from build123d import *

# Parameters (mm, degrees)
SKETCH1_R           = 1.85
SKETCH1_W           = 4.8
SKETCH1_H           = 4.8
BOSS_EXTRUDE1_DEPTH = 1.57
SKETCH2_W           = 4.8
SKETCH2_H           = 4.8
BOSS_EXTRUDE2_DEPTH = 1.47


with BuildPart() as part:
    # Sketch1 → Boss-Extrude1 (new body)
    # profile 1 of 2: a face of its own
    with BuildSketch(Plane(origin=(0, 0, 0), x_dir=(1, 0, 0), z_dir=(0, 1, 0))):
        with BuildLine():
            ThreePointArc((-11.5, 9.5), (-10.914213562, 10.914213562), (-9.5, 11.5))
            Line((-9.5, 11.5), (9.5, 11.5))
            ThreePointArc((9.5, 11.5), (10.914213562, 10.914213562), (11.5, 9.5))
            Line((11.5, 9.5), (11.5, -9.5))
            ThreePointArc((11.5, -9.5), (10.914213562, -10.914213562), (9.5, -11.5))
            Line((9.5, -11.5), (-9.5, -11.5))
            ThreePointArc((-9.5, -11.5), (-10.914213562, -10.914213562), (-11.5, -9.5))
            Line((-11.5, -9.5), (-11.5, 9.5))
        make_face()
        with Locations(Location((-8, -8, 0), (0, 0, 270))):
            Circle(SKETCH1_R, mode=Mode.SUBTRACT)
        with Locations(Location((8, -8, 0), (0, 0, 270))):
            Circle(SKETCH1_R, mode=Mode.SUBTRACT)
        with Locations(Location((8, 8, 0), (0, 0, 270))):
            Circle(SKETCH1_R, mode=Mode.SUBTRACT)
        with Locations(Location((-8, 8, 0), (0, 0, 270))):
            Circle(SKETCH1_R, mode=Mode.SUBTRACT)
        Rectangle(SKETCH1_W, SKETCH1_H, mode=Mode.SUBTRACT)
    # profile 2 of 2: a face of its own
    with BuildSketch(Plane(origin=(0, 0, 0), x_dir=(1, 0, 0), z_dir=(0, 1, 0))):
        Rectangle(SKETCH1_W, SKETCH1_H)
    extrude(amount=BOSS_EXTRUDE1_DEPTH)

    # Sketch2 → Boss-Extrude2 (add)
    with BuildSketch(Plane(origin=(0, 1.57, 0), x_dir=(1, 0, 0), z_dir=(0, 1, 0))):
        Rectangle(SKETCH2_W, SKETCH2_H)
    extrude(amount=BOSS_EXTRUDE2_DEPTH)


solid = part.part
Geometry check sheet. Reference: the model listing, model coordinates, mm. A direction names the side the tool comes from. Coordinates: 2 decimals unless noted, no trailing zeros. Order: outer loops, then holes, each group sorted by start corner. A loop starts at its lowest first (then second) coordinate and runs counter-clockwise, first axis right, second up. Notation, with made-up numbers: M 23,-11 L 39,-11 A28 ccw 39,23 Z; hole C 46.25,26 d4. An arc over 180 degrees is marked long. Use CSV: the item, a comma, the result in double quotes.
Item 1: Cross-section at D-D on x = 1.5. Record the cut outline in (y, z).
Returned:
outline,"M 0,-11.5 L 1.57,-11.5 L 1.57,-2.4 L 3.04,-2.4 L 3.04,2.4 L 1.57,2.4 L 1.57,11.5 L 0,11.5 Z"
Item 2: Tool access check on faces 4 (the flat face through (-2.4, 2, 0)), 5 (the flat face through (0, 2, -2.4)), 6 (the flat face through (0, 2, 2.4)), 7 (the flat face through (2.4, 2, 0)). Record the directions out of +Z, -Z, +X, -X, +Y, -Y that give a thin tool (end or side, any length) a straight path to the whole face; none if there is none.
Returned:
face 4,"+Z, -Z, -X, +Y"
face 5,"-Z, +X, -X, +Y"
face 6,"+Z, +X, -X, +Y"
face 7,"+Z, -Z, +X, +Y"
Item 3: Mould release check, pull along X, two halves, no side actions. Record for faces 1 (the cylindrical face through (6.874, 0.774, 6.532)), 2 (the flat face through (0, 1.57, -3)), 3 (the flat face through (-11.5, 1, 0)): pulls with the +X half, pulls with the -X half, needs draft (parallel to the pull), parting line crosses it, or undercut.
Returned:
face 1,"undercut"
face 2,"needs draft"
face 3,"pulls with the -X half"
Item 4: Cross-section at B-B on x = 8. Record the cut outline in (y, z), then the cut area to 3 significant figures.
Returned:
outline,"M 0,-11.5 L 1.57,-11.5 L 1.57,-9.85 L 0,-9.85 Z; M 0,-6.15 L 1.57,-6.15 L 1.57,6.15 L 0,6.15 Z; M 0,9.85 L 1.57,9.85 L 1.57,11.5 L 0,11.5 Z"
area,"24.5 mm2"
Item 5: Cross-section at C-C on y = 0.6. Record the cut outline in (x, z), then the cut area to 3 significant figures.
Returned:
outline,"M -11.5,-9.5 A2 ccw -9.5,-11.5 L 9.5,-11.5 A2 ccw 11.5,-9.5 L 11.5,9.5 A2 ccw 9.5,11.5 L -9.5,11.5 A2 ccw -11.5,9.5 Z; hole C -8,-8 d3.7; hole C -8,8 d3.7; hole C 8,-8 d3.7; hole C 8,8 d3.7"
area,"483 mm2"
Item 6: Thickness scan on line 1 along X through (y, z) = (1, 8); line 2 along X through (y, z) = (1.35, 9.25); line 3 along Y through (x, z) = (-8.5, 10). Record the ranges inside material, lowest first.
Returned:
line 1,"x = -11.5 to -9.85, -6.15 to 6.15, 9.85 to 11.5"
line 2,"x = -11.5 to -9.36, -6.64 to 6.64, 9.36 to 11.5"
line 3,"y = 0 to 1.57"
Item 7: Gauge pin test, flat ends, axial feed: pin 1 Ø5 at (x, z) = (8, -8) entering from +Y; pin 2 Ø8 at (x, z) = (-3.5, -6) entering from -Y; pin 3 Ø0.7 at (x, y) = (0, 2) entering from -Z; pin 4 Ø1.2 at (y, z) = (2.5, 0.5) entering from -X. Record the tip position at first contact, or that the pin passes through.
Returned:
pin 1,"stops at y = 1.57"
pin 2,"stops at y = 0"
pin 3,"stops at z = -2.4"
pin 4,"stops at x = -2.4"
Item 8: Cross-section at A-A on z = 8. Record the cut outline in (x, y).
Returned:
outline,"M -11.5,0 L -9.85,0 L -9.85,1.57 L -11.5,1.57 Z; M -6.15,0 L 6.15,0 L 6.15,1.57 L -6.15,1.57 Z; M 9.85,0 L 11.5,0 L 11.5,1.57 L 9.85,1.57 Z"
